Autodesk Inventor part; units mm, degrees
ref_plane "YZ Plane" through (0, 0, 0) normal (1, 0, 0) x (0, 1, 0)
ref_plane "XZ Plane" through (0, 0, 0) normal (0, 1, 0) x (-1, 0, 0)
ref_plane "XY Plane" through (0, 0, 0) normal (0, 0, 1) x (1, 0, 0)
sketch "Sketch1" plane through (0, 0, 0) normal (0, 0, 1) x (1, 0, 0)
  line L0 (139.9, -900) -> (139.9, 100) construction
  line L1 (-20.1001, -2.6887) -> (-20.0999, -902.6887) construction
  line L2 (139.9, -395.4887) -> (-20.1, -395.4887)
  line L3 (-20.1, -395.4887) -> (-20.1, -345.4887)
  line L4 (-20.1, -345.4887) -> (139.9, -345.4887)
  line L5 (139.9, -345.4887) -> (139.9, -395.4887)
  point P0 (0, 0)
  dimension "d0" = 50
extrude "Extrusion1" add sketch "Sketch1" along normal blind 4
fillet "Fillet1" radius 2 4 edges at (-20.1, -395.4887, 2) (-20.1, -345.4887, 2) (139.9, -395.4887, 2) (139.9, -345.4887, 2)
sketch "Sketch2" plane through (0, 0, 4) normal (0, 0, 1) x (1, 0, 0)
  line L0 (128.9999, 97.3113) -> (129.0001, -902.6887) construction
  line L1 (120.7999, 97.3113) -> (128.9999, 97.3113) construction
  line L2 (120.7999, 97.3113) -> (120.8001, -902.6887) construction
  line L3 (129.0001, -902.6887) -> (120.8001, -902.6887) construction
  line L4 (-1.0001, 97.3113) -> (-0.9999, -902.6887) construction
  line L5 (-9.2001, 97.3113) -> (-1.0001, 97.3113) construction
  line L6 (-9.2001, 97.3113) -> (-9.1999, -902.6887) construction
  line L7 (-0.9999, -902.6887) -> (-9.1999, -902.6887) construction
  line L8 (124.9001, -902.6887) -> (124.8999, 97.3113) construction
  line L9 (-5.1001, 97.3113) -> (-5.0999, -902.6887) construction
  circle A0 centre (51.3999, -385.9887) radius 1.5 construction
  circle A1 centre (20.3999, -385.9887) radius 1.5 construction
  circle A2 centre (20.3999, -354.9887) radius 1.5 construction
  circle A3 centre (51.3999, -354.9887) radius 1.5 construction
  circle A4 centre (124.9, -387.4887) radius 2
  circle A5 centre (124.9, -353.4887) radius 2
  circle A6 centre (51.3999, -385.9887) radius 1.5
  circle A7 centre (51.3999, -354.9887) radius 1.5
  circle A8 centre (20.3999, -354.9887) radius 1.5
  circle A9 centre (20.3999, -385.9887) radius 1.5
  circle A10 centre (-5.1, -387.4887) radius 2
  circle A11 centre (-5.1, -353.4887) radius 2
  line L10 (-18.1, -395.4887) -> (137.9, -395.4887)
  line L11 (137.9, -345.4887) -> (-18.1, -345.4887)
  point P0 (0, 0)
  dimension "d4" = 4
  dimension "d5" = 4
  dimension "d6" = 3
  dimension "d7" = 3
  dimension "d8" = 3
  dimension "d9" = 3
  dimension "d10" = 4
  dimension "d11" = 4
  dimension "d12" = 8
  dimension "d13" = 8
  dimension "d14" = 8
  dimension "d15" = 8
extrude "Extrusion2" cut sketch "Sketch2" against normal through all
properties part number "wiper motor holder"
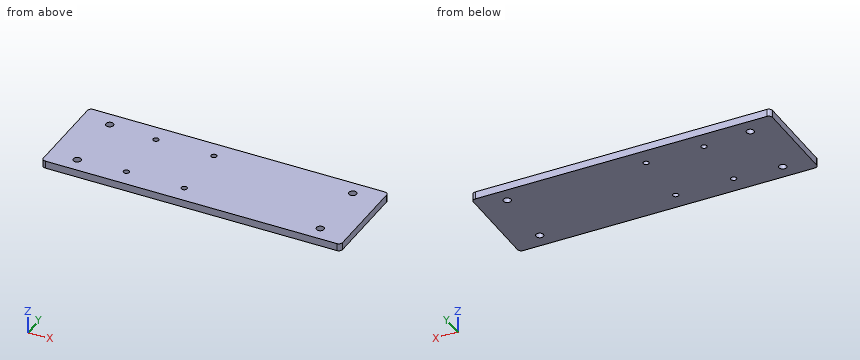
Source: CAD feature listing. Evaluate the final solid. Frame: model axes, mm. Round coordinates to 2 decimals unless told otherwise and drop trailing zeros. Loops run counter-clockwise (first coordinate to the right, second up) from the corner with the lowest first, then second, coordinate; pieces in that order, holes last. Notation, with made-up numbers: M 60.25,46.25 L 66.25,46.25 A23 cw 66.25,78.25 Z; hole C 42.25,47.25 d2. An arc over 180 degrees is marked long. Answer as CSV lines item,"result".
Q1. Contact query for flat-ended pins moving along their axis: pin 1 (2.5 mm diameter, centred on x = 124.9, y = -353.49, fed in from +Z); pin 2 (5 mm diameter, centred on x = 51.4, y = -385.99, fed in from +Z). Output: stop coordinate, or through.
Verdict:
pin 1,"passes through"
pin 2,"stops at z = 4"
Q2. Cut plane A-A (x = 124.9). Return the cut outline in (y, z), plus the area to 3 significant figures.
Verdict:
outline,"M -395.49,0 L -389.49,0 L -389.49,4 L -395.49,4 Z; M -385.49,0 L -355.49,0 L -355.49,4 L -385.49,4 Z; M -351.49,0 L -345.49,0 L -345.49,4 L -351.49,4 Z"
area,"168 mm^2"
Q3. Line query: line 1 along Y through (x, z) = (-5.1, 2.8); line 2 along X through (y, z) = (-387, 3.5); line 3 along X through (y, z) = (-386.5, 1). Output: solid intervals per line, ascending.
Verdict:
line 1,"y = -395.49 to -389.49, -385.49 to -355.49, -351.49 to -345.49"
line 2,"x = -20.1 to -7.04, -3.16 to 19.29, 21.51 to 50.29, 52.51 to 122.96, 126.84 to 139.9"
line 3,"x = -20.1 to -6.84, -3.36 to 18.99, 21.81 to 49.99, 52.81 to 123.16, 126.64 to 139.9"
